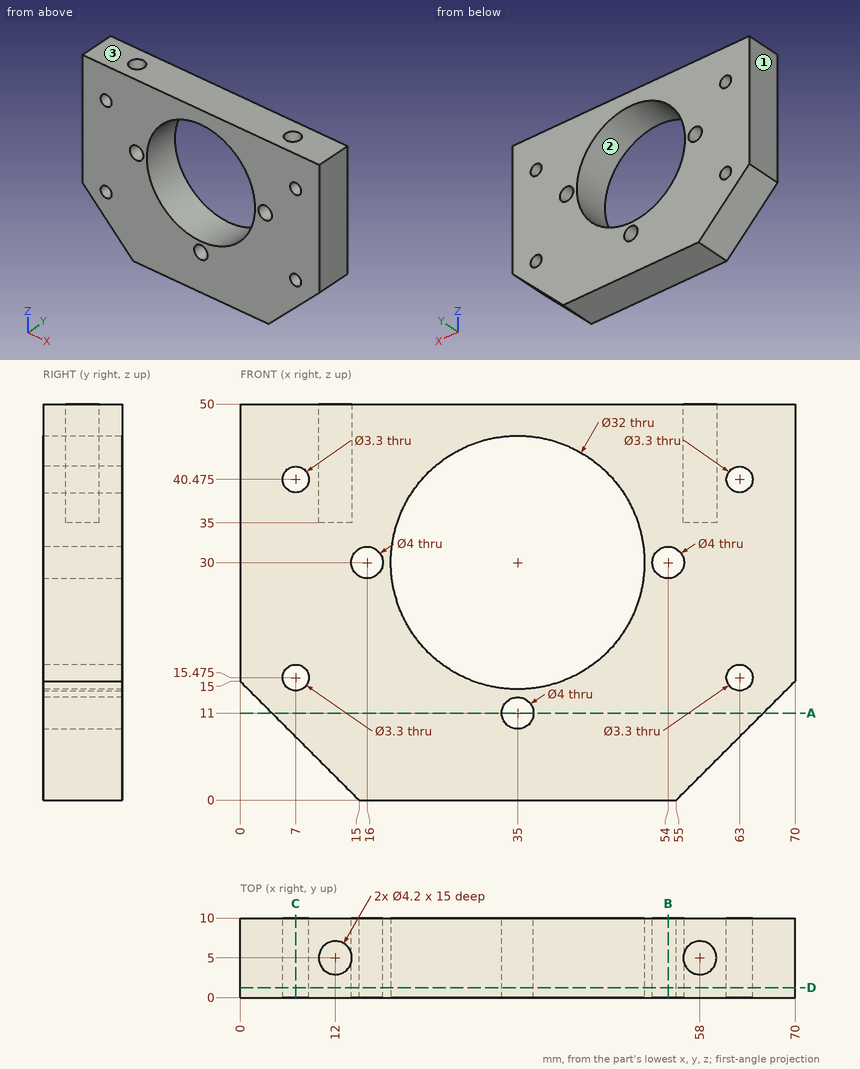
Geometry check sheet. Reference: drawing and pictorial views, mm from the part's lowest x, y, z. Round coordinates to 2 decimals unless told otherwise and drop trailing zeros. Write each loop counter-clockwise with the first axis right and the second up, starting at its lowest first coordinate (ties: lowest second). Pieces come first, ordered by that corner, then holes.
(1) Mould release check, pull along Z, two halves, no side actions. Record for the marked faces 1, 2 and 3: pulls with the +Z half, pulls with the -Z half, needs draft (parallel to the pull), parting line crosses it, or undercut.
Returned:
face 1: needs draft
face 2: undercut
face 3: pulls with the +Z half
(2) Section check D-D (y = 1.25). Give the number of separate pieces and of enclosed holes in the cut face, plus the area to 3 significant figures.
Returned:
separate pieces: 1
enclosed holes: 8
area: 2,400 mm2
(3) Material ranges on line 1 (X direction, y = 4.75, z = 30); line 2 (Y direction, x = 12, z = 43); line 3 (X direction, y = 9.75, z = 39.5), recorded low to high.
Returned:
line 1: x = 0 to 14, 18 to 19, 51 to 52, 56 to 70
line 2: y = 0 to 2.9, 7.1 to 10
line 3: x = 0 to 5.67, 8.33 to 22.13, 47.87 to 61.67, 64.33 to 70
(4) Section check B-B (x = 54). Enter the section's corners in (y, z), plus the area to 3 significant figures.
Returned:
outline: (0, 0) - (10, 0) - (10, 28) - (0, 28) - close; (0, 32) - (10, 32) - (10, 50) - (0, 50) - close
area: 460 mm2
(5) Section check A-A (z = 11). Enter the section's corners in (x, y), plus the area to 3 significant figures.
Returned:
outline: (4, 0) - (33, 0) - (33, 10) - (4, 10) - close; (37, 0) - (66, 0) - (66, 10) - (37, 10) - close
area: 580 mm2
(6) Depth check by flat-ended pin: pin 1 Ø2.5 at (x, z) = (16, 30) entering from +Y; pin 2 Ø1 at (x, y) = (61, 2.5) entering from -Z; pin 3 Ø2.5 at (x, y) = (12, 5) entering from +Z. Enter the tip coordinate at first touch or a pass-through.
Returned:
pin 1: passes through
pin 2: stops at z = 5.5
pin 3: stops at z = 35
(7) Section check C-C (x = 7). Enter the section's corners in (y, z) (3 decimals).
Returned:
outline: (0, 8) - (10, 8) - (10, 13.825) - (0, 13.825) - close; (0, 17.125) - (10, 17.125) - (10, 38.825) - (0, 38.825) - close; (0, 42.125) - (10, 42.125) - (10, 50) - (0, 50) - close
